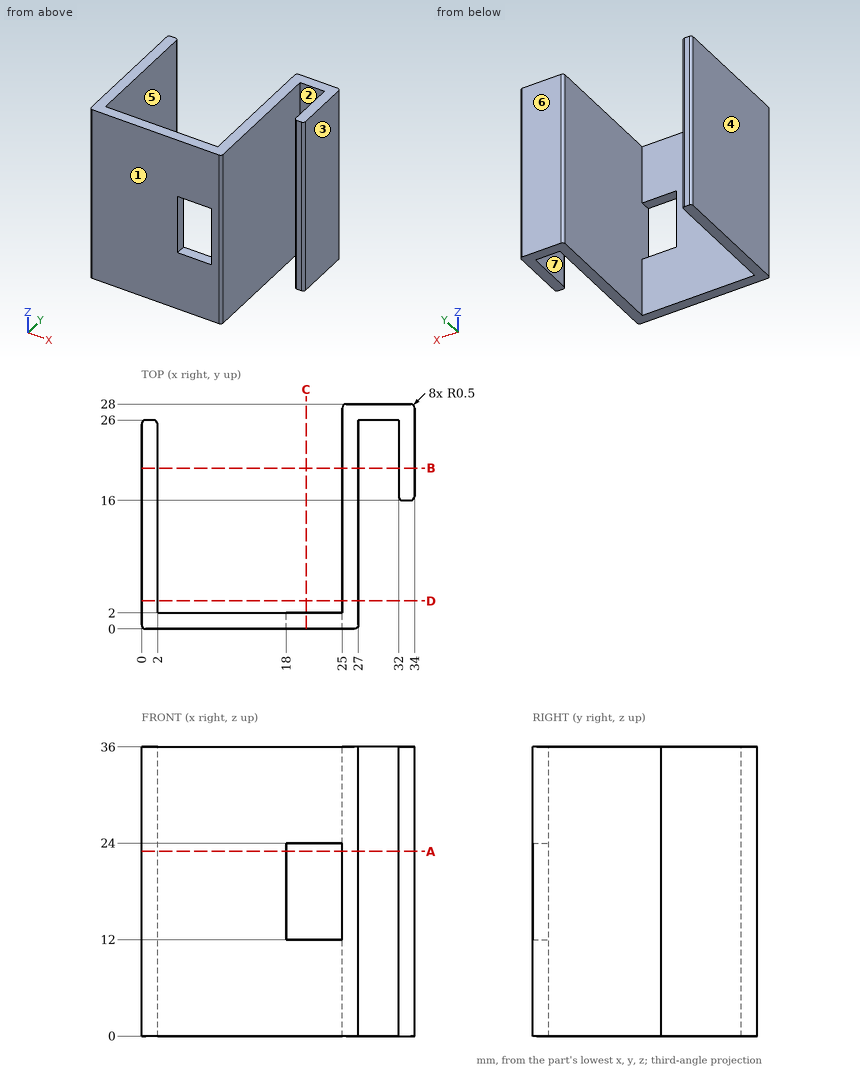
Could you check a few things on this drawing? It's one solid part, dimensions in mm from its lowest x, y, z. A direction names the side the tool comes from. Coordinates: 2 decimals unless noted, no trailing zeros. Order: outer loops, then holes, each group sorted by start corner. A loop starts at its lowest first (then second) coordinate and runs counter-clockwise, first axis right, second up.
1. If we section it at B-B (y = 20): Please give me the cut outline in (x, z).
2. If we section it at C-C (x = 20.5): Please give me the cut outline in (y, z), then the cut area to 3 significant figures.
3. If we section it at D-D (y = 3.5): Please give me the cut outline in (x, z).
4. If we section it at A-A (z = 23): Please give me the cut outline in (x, y), then the cut area to 3 significant figures.
5. For the marked faces 5, 6 and 7, which set-ups out of +Z, -Z, +X, -X, +Y, -Y let a thin tool reach every point of the face, with its end or its side?
6. I'm going to push flat-ended pins straight in: pin 1 (10 mm diameter, centred on x = 11, y = 9, fed in from +Z); pin 2 (1.6 mm diameter, centred on x = 21, y = 1, fed in from -Z); pin 3 (2.5 mm diameter, centred on x = 30, z = 20, fed in from -Y); pin 4 (0.6 mm diameter, centred on y = 0.5, z = 16.5, fed in from +X). Where does each tip first touch, or does it pass through?
7. Thinking about a two-plate mould opening in X: for the marked faces 1, 2, 3 and 4, which applies, +X half, -X half, draft (parallel to the pull), parting line (faces both ways), or undercut?
8. I need wall thicknesses on line 1 (X direction, y = 19.75, z = 21); line 2 (X direction, y = 16.25, z = 19); line 3 (X direction, y = 15.5, z = 18). Which ranges of each line are inside material? Lowest first, please.
Entries:
1. outline: (0, 0) - (2, 0) - (2, 36) - (0, 36) - close; (25, 0) - (27, 0) - (27, 36) - (25, 36) - close; (32, 0) - (34, 0) - (34, 36) - (32, 36) - close
2. outline: (0, 0) - (2, 0) - (2, 12) - (0, 12) - close; (0, 24) - (2, 24) - (2, 36) - (0, 36) - close
2. area: 48.0 mm2
3. outline: (0, 0) - (2, 0) - (2, 36) - (0, 36) - close; (25, 0) - (27, 0) - (27, 36) - (25, 36) - close
4. outline: (0, 0.5) arc R0.5 ccw to (0.5, 0) - (18, 0) - (18, 2) - (2, 2) - (2, 25.5) arc R0.5 ccw to (1.5, 26) - (0.5, 26) arc R0.5 ccw to (0, 25.5) - close; (25, 0) - (26.5, 0) arc R0.5 ccw to (27, 0.5) - (27, 26) - (32, 26) - (32, 16.5) arc R0.5 ccw to (32.5, 16) - (33.5, 16) arc R0.5 ccw to (34, 16.5) - (34, 27.5) arc R0.5 ccw to (33.5, 28) - (25.5, 28) arc R0.5 ccw to (25, 27.5) - close
4. area: 174 mm2
5. face 5: +Z, -Z, +Y
5. face 6: +Z, -Z, +X, -X, +Y
5. face 7: +Z, -Z, -Y
6. pin 1: passes through
6. pin 2: stops at z = 0
6. pin 3: stops at y = 26
6. pin 4: stops at x = 27
7. face 1: draft
7. face 2: undercut
7. face 3: +X half
7. face 4: -X half
8. line 1: x = 0 to 2, 25 to 27, 32 to 34
8. line 2: x = 0 to 2, 25 to 27, 32.07 to 33.93
8. line 3: x = 0 to 2, 25 to 27
